from build123d import *

# Parameters (mm, degrees)
F0_R     = 6.35
F1_DEPTH = 63.5
F3_R     = 9.525
F3_R_2   = 6.35
F4_DEPTH = 12.7
F2_R     = 9.525
F2_R_2   = 6.35
F5_DEPTH = 12.7


with BuildPart() as f1:
    # F0 (on Front) → F1 (new body, symmetric)
    with BuildSketch(Plane.XZ):
        Circle(F0_R)
    extrude(amount=F1_DEPTH, both=True)

    # F3 (on face) → F4 (join)
    with BuildSketch(Plane(origin=(0, 63.5, 0), x_dir=(-1, 0, 0), z_dir=(0, 1, 0))):
        Circle(F3_R)
        Circle(F3_R_2, mode=Mode.SUBTRACT)
    extrude(amount=-F4_DEPTH)

    # F2 (on face) → F5 (join)
    with BuildSketch(Plane.XZ.offset(63.5)):
        Circle(F2_R)
        Circle(F2_R_2, mode=Mode.SUBTRACT)
    extrude(amount=-F5_DEPTH)


solid = f1.part
Could you check a few things on this model? Use its own coordinates, in mm. A direction names the side the tool comes from. Coordinates: 2 decimals unless noted, no trailing zeros. Order: outer loops, then holes, each group sorted by start corner. A loop starts at its lowest first (then second) coordinate and runs counter-clockwise, first axis right, second up.
Q1. Suppose I cut it at B-B on z = 0. Please give me the cut outline in (x, y) (3 decimals).
Q2. Suppose I cut it at D-D on y = -48. Please give me the cut outline in (x, z), and give its area (3 significant figures).
Q3. Suppose I cut it at A-A on x = 0. Please give me the cut outline in (y, z) (3 decimals).
Q4. Suppose I cut it at C-C on z = 8.25. Please give me the cut outline in (x, y).
Q5. Which directions (+Z, -Z, +X, -X, +Y, -Y) give clear straight access to the entire face, cutting with the end or side of a thin tool? Please do faces 4 (the flat face through (0, 63.5, 0)), 5 (the cylindrical face through (-1.38, -0.71, -6.2)).
Q6. Please list where these lines run through material, in increasing order: L1, parallel to Y at x = 0, z = 8.25; L2, parallel to X at y = 7, z = -0.25.
Q7. Thinking about a two-plate mould opening in Y: for faces 1 (the flat face through (0, -63.5, 0)), 2 (the cylindrical face through (-7.559, -57.239, -5.796)), 3 (the flat face through (2, -50.8, -6.2)), which applies, released by +Y, released by -Y, zero draft, split by the parting line, or undercut?
Q8. Will these pins go through, and if not, where does the flat tip stop? pin 1 (6 mm diameter, centred on x = -4.5, y = 47.5, fed in from -Z); pin 2 (3 mm diameter, centred on y = -19.5, z = -4, fed in from -X); pin 3 (1.5 mm diameter, centred on x = 5.5, y = -14.5, fed in from +Z); pin 4 (1 mm diameter, centred on x = 7, y = 46.5, fed in from -Z).
Answer:
1. outline: (-9.525, -63.5) - (9.525, -63.5) - (9.525, -50.8) - (6.35, -50.8) - (6.35, 50.8) - (9.525, 50.8) - (9.525, 63.5) - (-9.525, 63.5) - (-9.525, 50.8) - (-6.35, 50.8) - (-6.35, -50.8) - (-9.525, -50.8) - close
2. outline: circle Ø12.7 at (0, 0)
2. area: 127 mm2
3. outline: (-63.5, -9.525) - (-50.8, -9.525) - (-50.8, -6.35) - (50.8, -6.35) - (50.8, -9.525) - (63.5, -9.525) - (63.5, 9.525) - (50.8, 9.525) - (50.8, 6.35) - (-50.8, 6.35) - (-50.8, 9.525) - (-63.5, 9.525) - close
4. outline: (-4.76, -63.5) - (4.76, -63.5) - (4.76, -50.8) - (-4.76, -50.8) - close; (-4.76, 50.8) - (4.76, 50.8) - (4.76, 63.5) - (-4.76, 63.5) - close
5. face 4: +Z, -Z, +X, -X, +Y
5. face 5: none
6. L1: y = -63.5 to -50.8, 50.8 to 63.5
6. L2: x = -6.35 to 6.35
7. face 1: released by -Y
7. face 2: zero draft
7. face 3: undercut
8. pin 1: stops at z = -6.17
8. pin 2: stops at x = -5.84
8. pin 3: stops at z = 4.21
8. pin 4: passes through
